from build123d import *

# Parameters (mm, degrees)
BOSS_EXTRU_1_DEPTH      = 60
ESQUISSE1_3_R           = 1.8
ESQUISSE1_3_R_2         = 7
BOSS_EXTRU_2_DEPTH      = 3
ENL_V_MAT_EXTRU_2_DEPTH = 50
ESQUISSE2_W             = 8
ESQUISSE2_H             = 8
ESQUISSE2_R             = 2.3
BOSS_EXTRU_4_DEPTH      = 6


with BuildPart() as part:
    # Esquisse1 → Boss.-Extru.1 (new body)
    with BuildSketch(Plane.XY):
        with BuildLine():
            ThreePointArc((18, 0), (12.727922061, -12.727922061), (0, -18))
            Line((0, -18), (18, -18))
            Line((18, -18), (18, 0))
        make_face()
        with BuildLine():
            ThreePointArc((0, -18), (-12.727922061, -12.727922061), (-18, 0))
            Line((-18, 0), (-18, -18))
            Line((-18, -18), (0, -18))
        make_face()
        with BuildLine():
            Line((-14, 0), (-18, 0))
            ThreePointArc((-18, 0), (-12.727922061, -12.727922061), (0, -18))
            ThreePointArc((0, -18), (12.727922061, -12.727922061), (18, 0))
            Line((18, 0), (14, 0))
            ThreePointArc((14, 0), (0, -14), (-14, 0))
        make_face()
    extrude(amount=-BOSS_EXTRU_1_DEPTH)

    # Esquisse1<3> → Boss.-Extru.2 (add)
    with BuildSketch(Plane.XY):
        with BuildLine():
            Line((-13, 18), (-18, 13))
            Line((-18, 13), (-18, 0))
            Line((-18, 0), (-14, 0))
            ThreePointArc((-14, 0), (0, -14), (14, 0))
            Line((14, 0), (18, 0))
            Line((18, 0), (18, 13))
            Line((18, 13), (13, 18))
            Line((13, 18), (-13, 18))
        make_face()
        with Locations((0, 10)):
            Circle(ESQUISSE1_3_R, mode=Mode.SUBTRACT)
        with Locations((0, -10)):
            Circle(ESQUISSE1_3_R, mode=Mode.SUBTRACT)
        with Locations((-10, 0)):
            Circle(ESQUISSE1_3_R, mode=Mode.SUBTRACT)
        Circle(ESQUISSE1_3_R_2, mode=Mode.SUBTRACT)
        with Locations((10, 0)):
            Circle(ESQUISSE1_3_R, mode=Mode.SUBTRACT)
    extrude(amount=-BOSS_EXTRU_2_DEPTH)

    # Esquisse3 → Enlèv. mat.-Extru.2 (cut)
    with BuildSketch(Plane.ZY.offset(18)):
        Polygon((-30, 0), (-20, 0), (-20, -13), (-40, -13), (-40, 0), align=None)
    extrude(amount=-ENL_V_MAT_EXTRU_2_DEPTH, mode=Mode.SUBTRACT)

    # Esquisse2 → Boss.-Extru.4 (add)
    # profile 1 of 4: a face of its own
    with BuildSketch(Plane.XZ.offset(18)):
        with Locations((22, -56)):
            Rectangle(ESQUISSE2_W, ESQUISSE2_H)
        with Locations(Location((22, -56, 0), (0, 0, 270))):
            Circle(ESQUISSE2_R, mode=Mode.SUBTRACT)
    # profile 2 of 4: a face of its own
    with BuildSketch(Plane.XZ.offset(18)):
        with Locations((-22, -56)):
            Rectangle(ESQUISSE2_W, ESQUISSE2_H)
        with Locations(Location((-22, -56, 0), (0, 0, 270))):
            Circle(ESQUISSE2_R, mode=Mode.SUBTRACT)
    # profile 3 of 4: a face of its own
    with BuildSketch(Plane.XZ.offset(18)):
        with Locations((-22, -4)):
            Rectangle(ESQUISSE2_W, ESQUISSE2_H)
        with Locations(Location((-22, -4, 0), (0, 0, 270))):
            Circle(ESQUISSE2_R, mode=Mode.SUBTRACT)
    # profile 4 of 4: a face of its own
    with BuildSketch(Plane.XZ.offset(18)):
        with Locations((22, -4)):
            Rectangle(ESQUISSE2_W, ESQUISSE2_H)
        with Locations(Location((22, -4, 0), (0, 0, 270))):
            Circle(ESQUISSE2_R, mode=Mode.SUBTRACT)
    extrude(amount=-BOSS_EXTRU_4_DEPTH)


solid = part.part
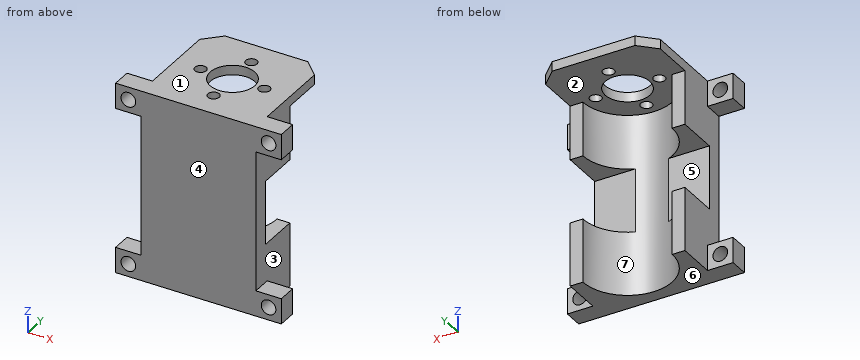
Verification items for the finished model (mm, model axes). Face numbers are marked on the shaded views. A direction names the side the tool comes from. Round coordinates to 2 decimals unless told otherwise and drop trailing zeros. Loops run counter-clockwise (first coordinate to the right, second up) from the corner with the lowest first, then second, coordinate; pieces in that order, holes last. Notation, with made-up numbers: (-14, 42.5) - (-10, 42.5) arc R26 cw to (-10, 69.5) - close; hole circle Ø8 at (-27, 5). An arc over 180 degrees is marked (long way). Write item = value, one per line.
Q1. Sectioned sample at C-C on x = 11. Record the boundary of the cut face in (y, z).
Here are the results:
outline = (-18, -60) - (-8.66, -60) - (-8.66, -40) - (-13, -40) - (-13, -20) - (-8.66, -20) - (-8.66, -3) - (-1.5, -3) - (-1.5, 0) - (-18, 0) - close; (1.5, -3) - (18, -3) - (18, 0) - (1.5, 0) - close
Q2. Tool access check on the marked faces 5, 6 and 7. Record the directions out of +Z, -Z, +X, -X, +Y, -Y that give a thin tool (end or side, any length) a straight path to the whole face; none if there is none.
Here are the results:
face_5 = +X, -X, +Y
face_6 = -Z, +X, -X, +Y, -Y
face_7 = -Z, +Y
Q3. Mould release check, pull along Z, two halves, no side actions. Record for the marked faces 1, 2, 3 and 4: +Z half, -Z half, draft (parallel to the pull), parting line (faces both ways), or undercut.
Here are the results:
face_1 = +Z half
face_2 = -Z half
face_3 = undercut
face_4 = draft
Q4. Material ranges on L1, parallel to X at y = -15.35, z = -4; L2, parallel to Y at x = 10, z = -2.4; L3, parallel to Z at x = -10.5, y = -11, recorded low to high.
Here are the results:
L1 = -26 to -24.3, -19.7 to 19.7, 24.3 to 26
L2 = -18 to -1.8, 1.8 to 18
L3 = -60 to -40, -20 to 0
Q5. Depth check by flat-ended pin: pin 1 (2 mm diameter, centred on x = 9.5, y = 1.5, fed in from -Z); pin 2 (2.5 mm diameter, centred on x = -22.5, z = -4, fed in from +Y); pin 3 (6 mm diameter, centred on x = -9.5, z = -42, fed in from +Y); pin 4 (3 mm diameter, centred on x = 16.5, z = -10, fed in from +Y). Enter the tip coordinate at first touch or a pass-through.
Here are the results:
pin_1 = -3
pin_2 = through
pin_3 = -6.3
pin_4 = 0
Q6. Sectioned sample at D-D on x = 0. Record the boundary of the cut face in (y, z), plus the area to 3 significant figures.
Here are the results:
outline = (-18, -60) - (-14, -60) - (-14, -3) - (-11.8, -3) - (-11.8, 0) - (-18, 0) - close; (-8.2, -3) - (-7, -3) - (-7, 0) - (-8.2, 0) - close; (7, -3) - (8.2, -3) - (8.2, 0) - (7, 0) - close; (11.8, -3) - (18, -3) - (18, 0) - (11.8, 0) - close
area = 272 mm^2
Q7. Sectioned sample at B-B on y = -4. Record the boundary of the cut face in (x, z), plus the area to 3 significant figures.
Here are the results:
outline = (-18, -60) - (-13.42, -60) - (-13.42, -40) - (-18, -40) - close; (-18, -20) - (-13.42, -20) - (-13.42, -3) - (-5.74, -3) - (-5.74, 0) - (-18, 0) - close; (5.74, -3) - (13.42, -3) - (13.42, -20) - (18, -20) - (18, 0) - (5.74, 0) - close; (13.42, -60) - (18, -60) - (18, -40) - (13.42, -40) - close
area = 413 mm^2
Q8. Sectioned sample at A-A on x = -22. Record the boundary of the cut face in (y, z), plus the area to 3 significant figures.
Here are the results:
outline = (-18, -60) - (-12, -60) - (-12, -58.3) - (-18, -58.3) - close; (-18, -53.7) - (-12, -53.7) - (-12, -52) - (-18, -52) - close; (-18, -8) - (-12, -8) - (-12, -6.3) - (-18, -6.3) - close; (-18, -1.7) - (-12, -1.7) - (-12, 0) - (-18, 0) - close
area = 40.8 mm^2
